from build123d import *

# Parameters (mm, degrees)
SKETCH1_R         = 137.941576563
EXTRUDE1_DEPTH    = 3.175
EXTRUDE3_DEPTH    = 4.175
SKETCH4_R         = 1.5875
EXTRUDE4_DEPTH    = 4.175
CIRPATTERN1_COUNT = 6


with BuildPart() as part:
    # Sketch1 → Extrude1 (new body)
    with BuildSketch(Plane(origin=(0, 0, 0), x_dir=(1, 0, 0), z_dir=(0, 1, 0))):
        with Locations(Location((0, 0, 0), (0, 0, 270))):  # turned: the seam where the file's is
            Circle(SKETCH1_R)
    extrude(amount=EXTRUDE1_DEPTH)

    # Sketch3 → Extrude3 (cut, through all)
    with BuildSketch(Plane(origin=(0, 3.175, 0), x_dir=(1, 0, 0), z_dir=(0, 1, 0))):
        with BuildLine():
            Line((25.204878031, -66.675), (107.95, -66.675))
            Line((107.95, -66.675), (107.95, 66.675))
            Line((107.95, 66.675), (25.204878031, 66.675))
            Line((25.204878031, 66.675), (25.204878031, 85.725))
            ThreePointArc((25.204878031, 85.725), (0.937561054, 109.992316976), (-23.329755922, 85.725))
            Line((-23.329755922, 85.725), (-26.9875, 66.675))
            Line((-26.9875, 66.675), (-107.95, 66.675))
            Line((-107.95, 66.675), (-107.95, -66.675))
            Line((-107.95, -66.675), (-26.9875, -66.675))
            Line((-26.9875, -66.675), (-23.329755922, -85.725))
            ThreePointArc((-23.329755922, -85.725), (0.937561054, -109.992316976), (25.204878031, -85.725))
            Line((25.204878031, -85.725), (25.204878031, -66.675))
        make_face()
    extrude(amount=-EXTRUDE3_DEPTH, mode=Mode.SUBTRACT)

    # Sketch4 → Extrude4 (cut, through all)
    with BuildSketch(Plane(origin=(0, 3.175, 0), x_dir=(-1, 0, 0), z_dir=(0, 1, 0))):
        with Locations(Location((120.65, 0, 0), (0, 0, 90))):  # turned: the seam where the file's is
            Circle(SKETCH4_R)
    extrude(amount=-EXTRUDE4_DEPTH, mode=Mode.SUBTRACT)

    # Sketch5 → CSK for #8 Flat Head Socket Cap Screw1 (revolve, cut)
    with BuildSketch(Plane(origin=(-120.65, 3.175, 0), x_dir=(0, 0, 1), z_dir=(1, 0, 0))):
        Polygon((0, 0), (0, 3.175), (2.2479, 3.175), (2.2479, 2.527474428), (4.445, 0), align=None)
    csk_for_8_flat_head_socket_cap_screw1 = revolve(axis=Axis((-120.65, 9.525, 0), (0, -1, 0)), mode=Mode.SUBTRACT)

    # CirPattern1: CSK for #8 Flat Head Socket Cap Screw1 ×6 about axis
    cirpattern1_axis = Axis((0, 0, 0), (0, 1, 0))
    for i in range(1, CIRPATTERN1_COUNT):
        add(csk_for_8_flat_head_socket_cap_screw1.rotate(cirpattern1_axis, i * 360 / CIRPATTERN1_COUNT), mode=Mode.SUBTRACT)


solid = part.part
Geometry: final body of the model. Coordinates: model frame, mm. A direction names the side the tool comes from. Give positions to 0.01 mm unless a question says otherwise; leave off trailing zeros. Loops run counter-clockwise (first coordinate to the right, second up) from the corner with the lowest first, then second, coordinate; pieces in that order, holes last. Notation, with made-up numbers: M -37.75,-35 L -13.75,-35 A10 cw -13.75,-27 Z; hole C 48.25,75 d5. An arc over 180 degrees is marked long. Put each result on its own line as item: value.
1) Material intervals for L1, parallel to X at y = 0.4, z = 0; L2, parallel to Z at x = -92.5, y = 1.2 (3 decimals); L3, parallel to Z at x = -91, y = 1.7 (3 decimals), sorted ascending. Write a range as from..to.
Computed values:
L1: x = -137.94..-122.9, -118.4..-107.95, 107.95..118.4, 122.9..137.94
L2: z = -102.331..-66.675, 66.675..102.331
L3: z = -103.667..-66.675, 66.675..103.667
2) Cut plane B-B, the plane x = -48. Return the cut outline in (y, z) (3 decimals).
Computed values:
outline: M 0,-129.321 L 3.175,-129.321 L 3.175,-66.675 L 0,-66.675 Z; M 0,66.675 L 3.175,66.675 L 3.175,129.321 L 0,129.321 Z
3) First-contact query: P1, Ø1.6, axis at y = 2.5, z = 7.5, coming from the -X side; P2, Ø5, axis at x = 60.33, z = -104.49, coming from the +Y side; P3, Ø1, axis at y = 2, z = 20, coming from the +X side. Flat tips, straight axial feed; report the tip coordinate or a pass-through.
Computed values:
P1: stops at x = -137.78
P2: stops at y = 0.94
P3: stops at x = 136.56
4) Reachability of faces 1 (the cylindrical face through (1.471, 1.61, -109.986)), 2 (the conical face through (-60.22, 0.806, 106.869)) from +Z, -Z, +X, -X, +Y, -Y: full face, straight path, thin tool, end or side. Return the list, or none.
Computed values:
face 1: +Y, -Y
face 2: +Y
5) Cut plane C-C, the plane y = 1.8. Give the number of separate pieces and of enclosed holes in the cut face, plus the area to 3 significant figures.
Computed values:
separate pieces: 1
enclosed holes: 7
area: 27,000 mm^2
6) Cut plane A-A, the plane z = -70.5. Return the cut outline in (x, y) (3 decimals).
Computed values:
outline: M -118.565,0 L -26.253,0 L -26.253,3.175 L -118.565,3.175 Z; M 25.205,0 L 118.565,0 L 118.565,3.175 L 25.205,3.175 Z
7) Mould query, pull axis X, two halves, no side actions, for faces 3 (the conical face through (61.24, 0.81, -102.28)), 4 (the cylindrical face through (-134.661, 1.565, -29.903)), 5 (the flat face through (-30, 3.175, 71)). Classes: released by +X, released by -X, zero draft, split by the parting line, or undercut.
Computed values:
face 3: undercut
face 4: split by the parting line
face 5: zero draft
